from build123d import *

# Parameters (mm, degrees)
SKETCH_1_W           = 50.28
SKETCH_1_H           = 34.2
SKETCH_1_W_2         = 30.28
SKETCH_1_H_2         = 14.2
EXTRUDE_1_DEPTH      = 12.25
SKETCH_4_W           = 13
SKETCH_4_H           = 13.91
EXTRUDE_1_2_DEPTH    = 74.82
SKETCH_5_W           = 13.91
SKETCH_5_H           = 16.23
EXTRUDE_2_DEPTH      = 16
SKETCH_7_R           = 25.25
SKETCH_7_R_2         = 15.25
EXTRUDE_2_2_DEPTH    = 16.23
SKETCH_15_R          = 1.91
CUT_EXTRUDE_6_DEPTH  = 97.964478439
SKETCH_16_W          = 13.91
SKETCH_16_H          = 16.23
EXTRUDE_4_DEPTH      = 10
SKETCH_17_R          = 1.91
CUT_EXTRUDE_7_DEPTH  = 102.16913771
SKETCH_18_W          = 49.344544624
SKETCH_18_H          = 6.125
CUT_EXTRUDE_8_DEPTH  = 105.840616652
SKETCH_19_W          = 34.2
SKETCH_19_H          = 6.125
CUT_EXTRUDE_9_DEPTH  = 10
SKETCH_21_R          = 1.91
CUT_EXTRUDE_10_DEPTH = 10
SKETCH_20_R          = 1.91
CUT_EXTRUDE_11_DEPTH = 10
FILLET_START         = -7.1
FILLET_1_DEPTH       = 14.2
FILLET_2_DEPTH       = 14.2
SKETCH_29_W          = 13.91
SKETCH_29_H          = 74.82
EXTRUDE_5_DEPTH      = 10
SKETCH_30_W          = 10
SKETCH_30_H          = 58.59
CUT_EXTRUDE_13_DEPTH = 102.16913771
SKETCH_32_W          = 34.2
SKETCH_32_H          = 5.745736365
EXTRUDE_6_DEPTH      = 10
SKETCH_33_W          = 107.115454733
SKETCH_33_H          = 42.36882751
CUT_EXTRUDE_14_DEPTH = 92.791032993


with BuildPart() as part:
    # 草圖1 → Extrude 1 (new body)
    with BuildSketch(Plane(origin=(0, 0, 0), x_dir=(1, 0, 0), z_dir=(0, 1, 0))):
        Rectangle(SKETCH_1_W, SKETCH_1_H)
        Rectangle(SKETCH_1_W_2, SKETCH_1_H_2, mode=Mode.SUBTRACT)
    extrude(amount=EXTRUDE_1_DEPTH)

    # 草圖4 → Extrude 1 2 (add)
    with BuildSketch(Plane.XZ):
        with Locations((18.64, 0)):
            Rectangle(SKETCH_4_W, SKETCH_4_H)
    extrude(amount=EXTRUDE_1_2_DEPTH)

    # 草圖5 → Extrude 2 (add)
    with BuildSketch(Plane.ZY.offset(-12.14)):
        with Locations((0, -66.705)):
            Rectangle(SKETCH_5_W, SKETCH_5_H)
    extrude(amount=EXTRUDE_2_DEPTH)

    # 草圖7 → Extrude 2 2 (add)
    with BuildSketch(Plane(origin=(3.626674765, -74.82, 0), x_dir=(1, 0, 0), z_dir=(0, -1, 0))):
        with Locations((-30.978154344, 0)):
            Circle(SKETCH_7_R)
        with Locations((-30.978154344, 0)):
            Circle(SKETCH_7_R_2, mode=Mode.SUBTRACT)
    extrude(amount=-EXTRUDE_2_2_DEPTH)

    # 草圖15 → 除料-伸長6 (cut, through all)
    with BuildSketch(Plane(origin=(0, 0, -6.955), x_dir=(-1, 0, 0), z_dir=(0, 0, -1))):
        with Locations((-4.530883248, -66.705)):
            Circle(SKETCH_15_R)
    extrude(amount=-CUT_EXTRUDE_6_DEPTH, mode=Mode.SUBTRACT)

    # 草圖16 → 填料-伸長4 (add)
    with BuildSketch(Plane(origin=(-60, 0, 0), x_dir=(0, 0, -1), z_dir=(1, 0, 0))):
        with Locations((0, -66.705)):
            Rectangle(SKETCH_16_W, SKETCH_16_H)
    extrude(amount=EXTRUDE_4_DEPTH)

    # 草圖17 → 除料-伸長7 (cut, through all)
    with BuildSketch(Plane(origin=(0, 0, -6.955), x_dir=(-1, 0, 0), z_dir=(0, 0, -1))):
        with Locations((55.812362827, -66.705)):
            Circle(SKETCH_17_R)
    extrude(amount=-CUT_EXTRUDE_7_DEPTH, mode=Mode.SUBTRACT)

    # 草圖18 → 除料-伸長8 (cut, through all)
    with BuildSketch(Plane(origin=(0, 0, -17.1), x_dir=(-1, 0, 0), z_dir=(0, 0, -1))):
        with Locations((0.467727688, 9.1875)):
            Rectangle(SKETCH_18_W, SKETCH_18_H)
    extrude(amount=-CUT_EXTRUDE_8_DEPTH, mode=Mode.SUBTRACT)

    # 草圖19 → 除料-伸長9 (cut)
    with BuildSketch(Plane.ZY.offset(-24.204544624)):
        with Locations((0, 9.1875)):
            Rectangle(SKETCH_19_W, SKETCH_19_H)
    extrude(amount=-CUT_EXTRUDE_9_DEPTH, mode=Mode.SUBTRACT)

    # 草圖21 → 除料-伸長10 (cut)
    with BuildSketch(Plane(origin=(0, 6.125, 0), x_dir=(1, 0, 0), z_dir=(0, 1, 0))):
        with Locations(Location((17.69, 0, 0), (0, 0, 270))):
            Circle(SKETCH_21_R)
    extrude(amount=-CUT_EXTRUDE_10_DEPTH, mode=Mode.SUBTRACT)

    # 草圖20 → 除料-伸長11 (cut)
    with BuildSketch(Plane(origin=(0, 6.125, 0), x_dir=(1, 0, 0), z_dir=(0, 1, 0))):
        with Locations(Location((-17.395, 0, 0), (0, 0, 270))):
            Circle(SKETCH_20_R)
    extrude(amount=-CUT_EXTRUDE_11_DEPTH, mode=Mode.SUBTRACT)

    # 圓角1: read off the stored shape, not the designer's step
    # 圓角1 outline → 圓角1 (cut)
    with BuildSketch(Plane.XY.offset(FILLET_START)):
        with BuildLine():
            add(Edge.make_bspline(
                [(-15.14, 0), (-21.974170252, 5.199829476), (-25.14, 5.745736365)],
                knots=[0, 0, 0, 0.664102345, 0.664102345, 0.664102345], degree=2, weights=[1, 2.223777218, 1.822127795]))
            Line((-15.14, 0), (-15.14, 6.125))
            Line((-15.14, 6.125), (-25.14, 6.125))
            Line((-25.14, 6.125), (-25.14, 5.745736365))
        make_face()
    extrude(amount=FILLET_1_DEPTH, mode=Mode.SUBTRACT)

    # 圓角2: read off the stored shape, not the designer's step
    # 圓角2 outline → 圓角2 (cut)
    with BuildSketch(Plane.XY.offset(FILLET_START)):
        with BuildLine():
            Line((15.14, 6.125), (15.14, 0))
            add(Edge.make_bspline(
                [(15.14, 0), (21.974170252, 5.199829476), (25.14, 5.745736365)],
                knots=[0, 0, 0, 0.664102345, 0.664102345, 0.664102345], degree=2, weights=[1, 2.223777218, 1.822127795]))
            Line((25.14, 5.745736365), (25.14, 6.125))
            Line((25.14, 6.125), (15.14, 6.125))
        make_face()
    extrude(amount=FILLET_2_DEPTH, mode=Mode.SUBTRACT)

    # 草圖29 → 填料-伸長5 (add)
    with BuildSketch(Plane(origin=(25.14, 0, 0), x_dir=(0, 0, -1), z_dir=(1, 0, 0))):
        with Locations((0, -37.41)):
            Rectangle(SKETCH_29_W, SKETCH_29_H)
    extrude(amount=EXTRUDE_5_DEPTH)

    # 草圖30 → 除料-伸長13 (cut, through all)
    with BuildSketch(Plane.XY.offset(6.955)):
        with Locations((17.14, -29.295)):
            Rectangle(SKETCH_30_W, SKETCH_30_H)
    extrude(amount=-CUT_EXTRUDE_13_DEPTH, mode=Mode.SUBTRACT)

    # 草圖32 → 填料-伸長6 (add)
    with BuildSketch(Plane(origin=(25.14, 0, 0), x_dir=(0, 0, -1), z_dir=(1, 0, 0))):
        with Locations((0, 2.872868182)):
            Rectangle(SKETCH_32_W, SKETCH_32_H)
    extrude(amount=EXTRUDE_6_DEPTH)

    # 草圖33 → 除料-伸長14 (cut, through all)
    with BuildSketch(Plane(origin=(0, -58.59, 0), x_dir=(1, 0, 0), z_dir=(0, 1, 0))):
        with Locations((-31.417727367, 21.184413755)):
            Rectangle(SKETCH_33_W, SKETCH_33_H)
    extrude(amount=-CUT_EXTRUDE_14_DEPTH, mode=Mode.SUBTRACT)


solid = part.part
Input: part model. Units: mm. Frame: model coordinates. A direction names the side the tool comes from. Give positions to 0.01 mm unless a question says otherwise; leave off trailing zeros. Order: outer loops, then holes, each group sorted by start corner. A loop starts at its lowest first (then second) coordinate and runs counter-clockwise, first axis right, second up. Notation, with made-up numbers: (77, 60.5) - (89, 60.5) arc R25 ccw to (89, 94.5) - close; hole circle Ø1 at (-10, -20.5). An arc over 180 degrees is marked (long way). Answer as a JSON object with one key per item and string values. Group by question number.
Q1. Cut plane D-D, the plane y = -16. Output: boundary loops of the cut face in (x, z) (3 decimals).
Q2. Cut plane B-B, the plane z = -8.5. Output: boundary loops of the cut face in (x, y) (3 decimals), then the cut area to 3 significant figures.
Q3. Line query: probe 1 along X at (y, z) = (1.5, 0) (3 decimals); probe 2 along Y at (x, z) = (-8, 14) (3 decimals); probe 3 along Y at (x, z) = (-39, 15). Output: solid intervals per line, ascending.
Q4. Mould query, pull axis X, two halves, no side actions, for faces 6 (the face through (-25.14, 3, 0)), 7 (the face through (4.78, -64.81, 3.43)), 8 (the face through (-13, -74.82, 9)). Classes: pulls with the +X half, pulls with the -X half, needs draft (parallel to the pull), parting line crosses it, or undercut.
Q5. First-contact query: pin 1 Ø5 at (x, y) = (20.5, -47.5) entering from -Z (3 decimals); pin 2 Ø2 at (x, z) = (-50, 2) entering from +Y; pin 3 Ø6.5 at (y, z) = (2, 5.5) entering from -X. Flat tips, straight axial feed; report the tip coordinate or a pass-through.
Q6. Set-up query: faces 1 (the face through (-26.895, -66.819, 25.246)), 2 (the face through (30, 5.746, 0)), 3 (the face through (-27.016, -66.819, 15.246)), 4 (the face through (-20, -58.59, 16)), 5 (the face through (24, -46, 6.955)). Return all of +Z, -Z, +X, -X, +Y, -Y with unobstructed straight access to the full face (end or side cutting, diameter ignored); none if empty.
Q7. Cut plane C-C, the plane x = 27. Output: boundary loops of the cut face in (y, z) (3 decimals), then the cut area to 3 significant figures.
Q8. Cut plane A-A, the plane y = -60.5. Output: boundary loops of the cut face in (x, z) (3 decimals).
Results:
{
 "1": {"outline": "(22.14, -6.955) - (35.14, -6.955) - (35.14, 6.955) - (22.14, 6.955) - close"},
 "2": {"outline": "(-25.14, 0) - (35.14, 0) - (35.14, 5.746) - (25.14, 5.746) - (25.14, 6.125) - (-25.14, 6.125) - close", "area": "365 mm^2"},
 "3": {"probe 1": "-25.14 to -19.305, 19.6 to 35.14", "probe 2": "-74.82 to -58.59, 0 to 6.125", "probe 3": "-74.82 to -58.59"},
 "4": {"face 6": "pulls with the -X half", "face 7": "undercut", "face 8": "needs draft"},
 "5": {"pin 1": "z = -6.955", "pin 2": "y = -58.59", "pin 3": "x = -25.14"},
 "6": {"face 1": "+Z, -Y", "face 2": "+Z, -Z, +X, +Y", "face 3": "-Z, -Y", "face 4": "+Z, -Z, -X", "face 5": "+Z, +X, -Y"},
 "7": {"outline": "(-74.82, -6.955) - (0, -6.955) - (0, -17.1) - (5.746, -17.1) - (5.746, 17.1) - (0, 17.1) - (0, 6.955) - (-74.82, 6.955) - close", "area": "1,240 mm^2"},
 "8": {"outline": "(-60, 0) - (-42.601, 0) arc R15.25 cw to (-12.101, 0) - (22.14, 0) - (22.14, -6.955) - (35.14, -6.955) - (35.14, 6.955) - (-3.078, 6.955) arc R25.25 ccw to (-51.625, 6.955) - (-60, 6.955) - close"}
}
